Model file for the job. Use its own axes, mm. Give positions to 0.01 mm unless a question says otherwise; leave off trailing zeros. Write each loop counter-clockwise with the first axis right and the second up, starting at its lowest first coordinate (ties: lowest second). Pieces come first, ordered by that corner, then holes. Notation, with made-up numbers: (48, 61.25) - (67, 61.25) arc R32 ccw to (67, 100.25) - close; hole circle Ø5 at (32, 86.5). An arc over 180 degrees is marked (long way). Use a Markdown table: item, result. Add a question column.
```python
from build123d import *

# Parameters (mm, degrees)
BOSS_EXTRUDE1_DEPTH = 76.2
SKETCH7_R           = 7.5
CUT_EXTRUDE1_DEPTH  = 179


with BuildPart() as part:
    # Sketch1 → Boss-Extrude1 (new body)
    with BuildSketch(Plane(origin=(0, 0, 0), x_dir=(1, 0, 0), z_dir=(0, 1, 0))):
        with BuildLine():
            Line((-630.021699517, -47.499985829), (-630.021699517, -62.499985829))
            ThreePointArc((-630.021699517, -62.499985829), (0, -178), (630.021699517, -62.499985829))
            Line((630.021699517, -62.499985829), (630.021699517, -47.499985829))
            ThreePointArc((630.021699517, -47.499985829), (0, -163), (-630.021699517, -47.499985829))
        make_face()
    extrude(amount=BOSS_EXTRUDE1_DEPTH)

    # Sketch7 → Cut-Extrude1 (cut, through all)
    with BuildSketch(Plane.XY):
        with Locations((0, 38.1)):
            Circle(SKETCH7_R)
    extrude(amount=CUT_EXTRUDE1_DEPTH, mode=Mode.SUBTRACT)


solid = part.part
```
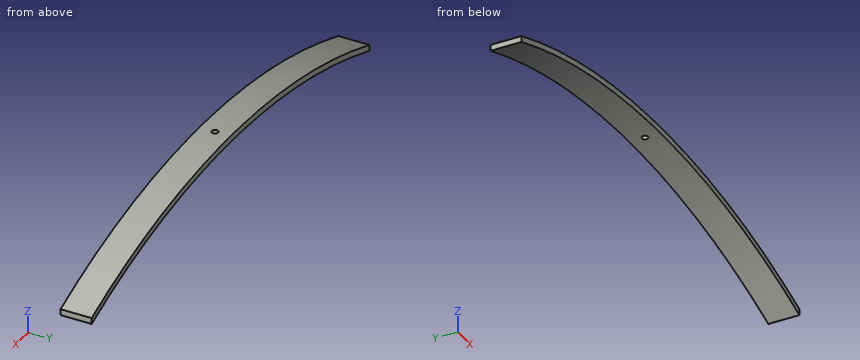
(1) Probe probe 1 along Y at (x, z) = (0, 166.5); probe 2 along Z at (x, y) = (210, 8); probe 3 along Z at (x, y) = (18, 40). List the from-to ranges inside material, lowest first. Write a range as [from, to].
(2) Band-saw the part on B-B (x = 69). Write the cut outline in (y, z), then the cut area to 3 significant figures.
(3) Flat gauge pins, fed straight in: pin 1 (1 mm diameter, centred on x = 107, y = 58.5, fed in from +Z); pin 2 (12 mm diameter, centred on x = 231, z = 161, fed in from -Y); pin 3 (12 mm diameter, centred on x = 481.5, y = 58, fed in from -Z); pin 4 (6 mm diameter, centred on x = 217, y = 28.5, fed in from +Z). Where does each tip first touch, or does it go through?
Model answer:
| question | item | result |
|---|---|---|
| 1 | probe 1 | y = [0, 30.6], [45.6, 76.2] |
| 1 | probe 2 | z = [150.54, 165.54] |
| 1 | probe 3 | z = [162.91, 177.91] |
| 2 | outline | (0, 161.66) - (76.2, 161.66) - (76.2, 176.66) - (0, 176.66) - close |
| 2 | area | 1,140 mm^2 |
| 3 | pin 1 | stops at z = 174.8 |
| 3 | pin 2 | stops at y = 0 |
| 3 | pin 3 | stops at z = 94.78 |
| 3 | pin 4 | stops at z = 165.06 |
